Autodesk Inventor part; units mm, degrees
ref_plane "YZ Plane" through (0, 0, 0) normal (1, 0, 0) x (0, 1, 0)
ref_plane "XZ Plane" through (0, 0, 0) normal (0, 1, 0) x (-1, 0, 0)
ref_plane "XY Plane" through (0, 0, 0) normal (0, 0, 1) x (1, 0, 0)
sketch "Sketch1" plane through (0, 0, 0) normal (1, 0, 0) x (0, 1, 0)
  line L0 (0, 0) -> (76.2, 0)
  line L1 (76.2, 0) -> (76.2, 50.8)
  line L2 (76.2, 50.8) -> (0, 50.8)
  line L3 (0, 50.8) -> (0, 0)
  line L4 (0, 25.4) -> (76.2, 25.4) construction
  circle A0 centre (25.4, 25.4) radius 3.81
  line L5 (43.5104, 25.4) -> (19.7104, 25.4) construction
  line L6 (19.7104, 19.7) -> (19.7104, 31.1)
  line L7 (19.7104, 31.1) -> (43.5104, 31.1)
  line L8 (43.5104, 31.1) -> (43.5104, 19.7)
  line L9 (43.5104, 19.7) -> (19.7104, 19.7)
  line L10 (31.6104, 19.7) -> (31.6104, 31.1) construction
  circle A1 centre (17.6022, 25.4) radius 1
  circle A2 centre (45.6186, 25.4) radius 1
  line L11 (25.4, 19.7) -> (25.4, 31.1) construction
  dimension "d0" = 76.2
  dimension "d1" = 50.8
  dimension "d2" = 23.8
  dimension "d3" = 11.4
  dimension "d4" = 2
  dimension "d5" = 2.1082
  dimension "d6" = 5.6896
  dimension "d7" = 25.4
extrude "Extrusion1" add sketch "Sketch1" along normal blind 5.08 contours L3 L2 L1 L0
properties part number "gripper_servo"
Build history of the part. All positions in model axes, mm. A direction names the side the tool comes from. Coordinates: 2 decimals unless noted, no trailing zeros. Order: outer loops, then holes, each group sorted by start corner. A loop starts at its lowest first (then second) coordinate and runs counter-clockwise, first axis right, second up. Notation, with made-up numbers: (-32.5, 71.25) - (8.5, 71.25) arc R32 ccw to (8.5, 100.25) - close; hole circle Ø2 at (-25.5, 34.5). An arc over 180 degrees is marked (long way). Write each question's results on one line, items separated by ' | '. Start each with the question number.
Item 1: Band-saw the part on C-C on z = 25.4. Write the cut outline in (x, y), and give its area (3 significant figures).
Item 2: Band-saw the part on B-B on x = 3.55. Write the cut outline in (y, z), and give its area (3 significant figures).
Item 3: Tool access for faces 5 (the face through (3, 32, 19.7)), 6 (the face through (3, 38, 0)): list every direction of +Z, -Z, +X, -X, +Y, -Y with a clear straight run to the whole face (end or side of a thin tool).
Item 4: Wall check: probe 1 along Y at (x, z) = (4, 26.5); probe 2 along Z at (x, y) = (1.45, 29); probe 3 along Z at (x, y) = (4.75, 17). Give the ranges that are in metal, low to high. Write a range as [from, to].
Item 5: Band-saw the part on A-A on y = 20.5. Write the cut outline in (x, z), and give its area (3 significant figures).
Item 6: Mould opens along Y. For faces 1 (the face through (3, 76.2, 25)), 2 (the face through (3, 43.51, 25)), 3 (the face through (3, 0, 26)), 4 (the face through (0, 37.6, 31.4)) say: released by +Y, released by -Y, zero draft, split by the parting line, or undercut.
Numbers:
1) outline: (0, 0) - (5.08, 0) - (5.08, 16.6) - (0, 16.6) - close; (0, 18.6) - (5.08, 18.6) - (5.08, 19.71) - (0, 19.71) - close; (0, 43.51) - (5.08, 43.51) - (5.08, 44.62) - (0, 44.62) - close; (0, 46.62) - (5.08, 46.62) - (5.08, 76.2) - (0, 76.2) - close | area: 246 mm^2
2) outline: (0, 0) - (76.2, 0) - (76.2, 50.8) - (0, 50.8) - close; hole circle Ø2 at (17.6, 25.4); hole (19.71, 19.7) - (43.51, 19.7) - (43.51, 31.1) - (19.71, 31.1) - close; hole circle Ø2 at (45.62, 25.4) | area: 3,590 mm^2
3) face 5: +X, -X | face 6: -Z, +X, -X, +Y, -Y
4) probe 1: [0, 19.71], [43.51, 76.2] | probe 2: [0, 19.7], [31.1, 50.8] | probe 3: [0, 24.6], [26.2, 50.8]
5) outline: (0, 0) - (5.08, 0) - (5.08, 19.7) - (0, 19.7) - close; (0, 31.1) - (5.08, 31.1) - (5.08, 50.8) - (0, 50.8) - close | area: 200 mm^2
6) face 1: released by +Y | face 2: undercut | face 3: released by -Y | face 4: zero draft
